from build123d import *

# Parameters (mm, degrees)
F0_R      = 20
F1_DEPTH  = 60
F2_R      = 10
F3_DEPTH  = 15
F4_DEPTH  = 45
F6_DEPTH  = 15
F8_DEPTH  = 5
F9_R      = 8
F10_DEPTH = 15.001


with BuildPart() as f1:
    # F0 (on Top) → F1 (new body)
    with BuildSketch(Plane.XY):
        with BuildLine():
            ThreePointArc((-29.580399, -5), (2.508788, -29.894916), (30, 0))
            ThreePointArc((30, 0), (2.508788, 29.894916), (-29.580399, 5))
            ThreePointArc((-29.580399, 5), (-30, 0), (-29.580399, -5))
        make_face()
        Circle(F0_R, mode=Mode.SUBTRACT)
    extrude(amount=-F1_DEPTH)

    # F2 (on face) → F3 (join)
    with BuildSketch(Plane(origin=(0, 0, -60), x_dir=(1, 0, 0), z_dir=(0, 0, -1))):
        with BuildLine():
            Line((16.583124, -25), (75, -25))
            ThreePointArc((75, -25), (100, 0), (75, 25))
            Line((75, 25), (16.583124, 25))
            ThreePointArc((16.583124, 25), (26.43382, 14.186372), (30, 0))
            ThreePointArc((30, 0), (26.43382, -14.186372), (16.583124, -25))
        make_face()
        with Locations((75, 0)):
            Circle(F2_R, mode=Mode.SUBTRACT)
    extrude(amount=-F3_DEPTH)

    # F0 (on Top) → F4 (join)
    with BuildSketch(Plane.XY):
        with BuildLine():
            ThreePointArc((-29.580399, -5), (-30, 0), (-29.580399, 5))
            Line((-29.580399, 5), (-60, 5))
            Line((-60, 5), (-60, 30))
            Line((-60, 30), (-74.087851, 30))
            Line((-74.087851, 30), (-75, 30))
            Line((-75, 30), (-75, 0))
            Line((-75, 0), (-75, -30))
            Line((-75, -30), (-60, -30))
            Line((-60, -30), (-60, -5))
            Line((-60, -5), (-29.580399, -5))
        make_face()
    extrude(amount=-F4_DEPTH)

    # F5 (on face) → F6 (join)
    with BuildSketch(Plane(origin=(0, 0, -45), x_dir=(1, 0, 0), z_dir=(0, 0, -1))):
        with BuildLine():
            Line((0, 30), (-60, 30))
            Line((-60, 30), (-60, -30))
            Line((-60, -30), (0, -30))
            ThreePointArc((0, -30), (-30, 0), (0, 30))
        make_face()
    extrude(amount=-F6_DEPTH)

    # F7 (on Front) → F8 (join, symmetric)
    with BuildSketch(Plane.XZ):
        Polygon((29.172541, 0), (29.172541, -43.929927), (54.172541, -43.929927), align=None)
    extrude(amount=F8_DEPTH, both=True)

    # F9 (on face) → F10 (cut, through all)
    with BuildSketch(Plane.YZ.offset(-60)):
        with Locations((-15, -15)):
            Circle(F9_R)
        with Locations((15, -15)):
            Circle(F9_R)
    extrude(amount=-F10_DEPTH, mode=Mode.SUBTRACT)


solid = f1.part
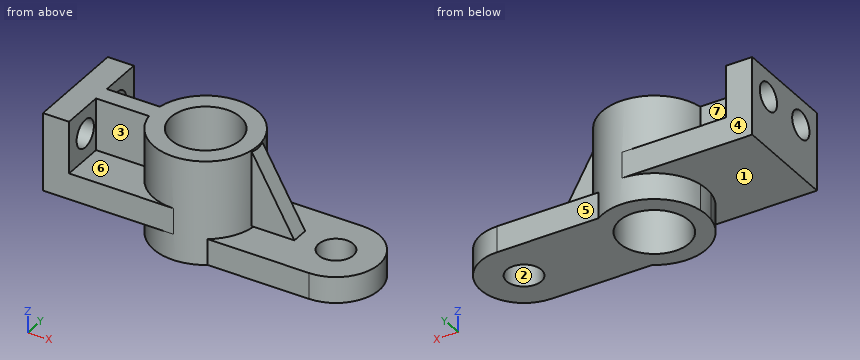
Input: part model. Units: mm. Frame: model coordinates. Face numbers are marked on the shaded views. A direction names the side the tool comes from. Give positions to 0.01 mm unless a question says otherwise; leave off trailing zeros. Loops run counter-clockwise (first coordinate to the right, second up) from the corner with the lowest first, then second, coordinate; pieces in that order, holes last. Notation, with made-up numbers: M -28.75,-9 L -2.75,-9 A18 ccw -2.75,0 Z; hole C 33,-28.5 d1. An arc over 180 degrees is marked long. Use one line per item in the form item = value.
1. Pull-direction query (Y, two-part tool) for the marked faces 1, 2, 3 and 4; classes: released by +Y, released by -Y, zero draft, split by the parting line, or undercut.
Numbers:
face_1 = zero draft
face_2 = undercut
face_3 = released by -Y
face_4 = released by +Y
2. Reachability of the marked faces 5, 6 and 7 from +Z, -Z, +X, -X, +Y, -Y: full face, straight path, thin tool, end or side. Return the list, or none.
Numbers:
face_5 = +Z, -Z, +X, +Y
face_6 = +Z, -Y
face_7 = +Z, +Y
3. Section query A-A, the plane y = 15. Return the cut outline in (x, z).
Numbers:
outline = M -75,-45 L -25.98,-45 L -25.98,-60 L -13.23,-60 L -13.23,0 L -25.98,0 L -25.98,-30 L -60,-30 L -60,-23 L -75,-23 Z; M -75,-7 L -60,-7 L -60,0 L -75,0 Z; M 13.23,-60 L 95,-60 L 95,-45 L 25.98,-45 L 25.98,0 L 13.23,0 Z
4. Line query: L1, parallel to Z at x = -64, y = 15; L2, parallel to Y at x = 75, z = -56; L3, parallel to X at y = -6, z = -6.5. Output: solid intervals per line, ascending.
Numbers:
L1 = -45 to -23, -7 to 0
L2 = -25 to -10, 10 to 25
L3 = -75 to -60, -29.39 to -19.08, 19.08 to 29.39
5. Section query C-C, the plane z = -38.5. Return the cut outline in (x, y).
Numbers:
outline = M -75,-30 L 0,-30 A30 ccw 29.58,-5 L 51.08,-5 L 51.08,5 L 29.58,5 A30 ccw 0,30 L -75,30 Z; hole C 0,0 d40
6. First-contact query: pin 1 (14.5 mm diameter, centred on y = -15, z = -15, fed in from +X); pin 2 (7.5 mm diameter, centred on x = 37, z = -51.5, fed in from +Y); pin 3 (18 mm diameter, centred on x = -47, y = 4.5, fed in from -Z); pin 4 (18 mm diameter, centred on x = 75, y = 0, fed in from +Z). Flat tips, straight axial feed; report the tip coordinate or a pass-through.
Numbers:
pin_1 = 28.98
pin_2 = 25
pin_3 = -45
pin_4 = through
7. Section query B-B, the plane x = 2. Return the cut outline in (y, z).
Numbers:
outline = M -29.93,-60 L -19.9,-60 L -19.9,0 L -29.93,0 Z; M 19.9,-60 L 29.93,-60 L 29.93,0 L 19.9,0 Z
8. Section query D-D, the plane x = -45.5. Return the cut outline in (y, z).
Numbers:
outline = M -30,-45 L 30,-45 L 30,-30 L 5,-30 L 5,0 L -5,0 L -5,-30 L -30,-30 Z
